Check sheet for the modelled part. Datum: model origin and axes. Units: mm. Give positions to 0.01 mm unless a question says otherwise; leave off trailing zeros. Loops run counter-clockwise (first coordinate to the right, second up) from the corner with the lowest first, then second, coordinate; pieces in that order, holes last. Notation, with made-up numbers: (63, -3) -> (95, -3) arc R23 ccw to (95, 8) -> close; hole circle Ø9 at (58, 40.5). An arc over 180 degrees is marked (long way). Write each question's results on one line, items separated by ' | '. Start each with the question number.
Item 1: Cross-section at A-A on z = 0. Enter the section's corners in (x, y), then the cut area to 3 significant figures.
Item 2: Cross-section at B-B on y = 4. Enter the section's corners in (x, z), then the cut area to 3 significant figures.
Item 3: Gauge pin test, flat end, axial feed: pin 1 Ø1.5 at (x, z) = (3.5, -1) entering from +Y. Record the tip position at first contact, or that the pin passes through.
Item 4: Cross-section at C-C on x = 30. Enter the section's corners in (y, z).
Item 5: Scan lines: line 1 along X through (y, z) = (5.25, -0.8); line 2 along Z through (x, y) = (-6.5, 0.25); line 3 along X through (y, z) = (4.5, -0.3). Record each from-to range of solid material in increasing order.
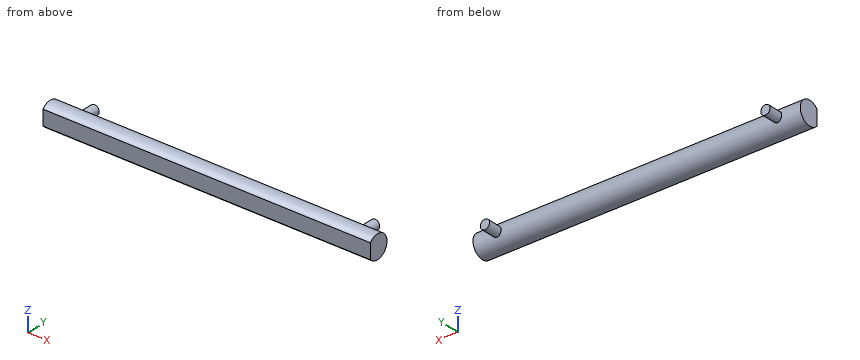
from build123d import *

# Parameters (mm, degrees)
F0_R     = 2.5
F1_DEPTH = 35
F2_R     = 1
F3_DEPTH = 5.5
F5_DEPTH = 70.0010001


with BuildPart() as f1:
    # F0 (on Right) → F1 (new body, symmetric)
    with BuildSketch(Plane.YZ):
        Circle(F0_R)
    extrude(amount=F1_DEPTH, both=True)

    # F2 (on Front) → F3 (join)
    with BuildSketch(Plane.XZ):
        with Locations((-30, 0)):
            Circle(F2_R)
        with Locations((30, 0)):
            Circle(F2_R)
    extrude(amount=-F3_DEPTH)

    # F4 (on face) → F5 (cut, through all)
    with BuildSketch(Plane.YZ.offset(35)):
        with BuildLine():
            Line((-1.9, -1.6248076809), (-1.9, 1.6248076809))
            ThreePointArc((-1.9, 1.6248076809), (-2.5, 0), (-1.9, -1.6248076809))
        make_face()
    extrude(amount=-F5_DEPTH, mode=Mode.SUBTRACT)


solid = f1.part
Answer sheet:
1) outline: (-35, -1.9) -> (35, -1.9) -> (35, 2.5) -> (31, 2.5) -> (31, 5.5) -> (29, 5.5) -> (29, 2.5) -> (-29, 2.5) -> (-29, 5.5) -> (-31, 5.5) -> (-31, 2.5) -> (-35, 2.5) -> close | area: 320 mm²
2) outline: circle Ø2 at (-30, 0); circle Ø2 at (30, 0) | area: 6.28 mm²
3) pin 1: stops at y = 2.49
4) outline: (-1.9, -1.62) arc R2.5 ccw to (2.29, -1) -> (5.5, -1) -> (5.5, 1) -> (2.29, 1) arc R2.5 ccw to (-1.9, 1.62) -> close
5) line 1: x = -30.6 to -29.4, 29.4 to 30.6 | line 2: z = -2.49 to 2.49 | line 3: x = -30.95 to -29.05, 29.05 to 30.95
